Part print with two shaded views. Sizes in mm from the minimum x, y, z corner. A direction names the side the tool comes from. Round coordinates to 2 decimals unless told otherwise and drop trailing zeros. Order: outer loops, then holes, each group sorted by start corner. A loop starts at its lowest first (then second) coordinate and runs counter-clockwise, first axis right, second up. Notation, with made-up numbers: (83, 57) -> (90, 57) arc R26 cw to (90, 78) -> close; hole circle Ø4 at (20.25, -9.75). An arc over 180 degrees is marked (long way). Answer as a JSON object with one key per item and string values.
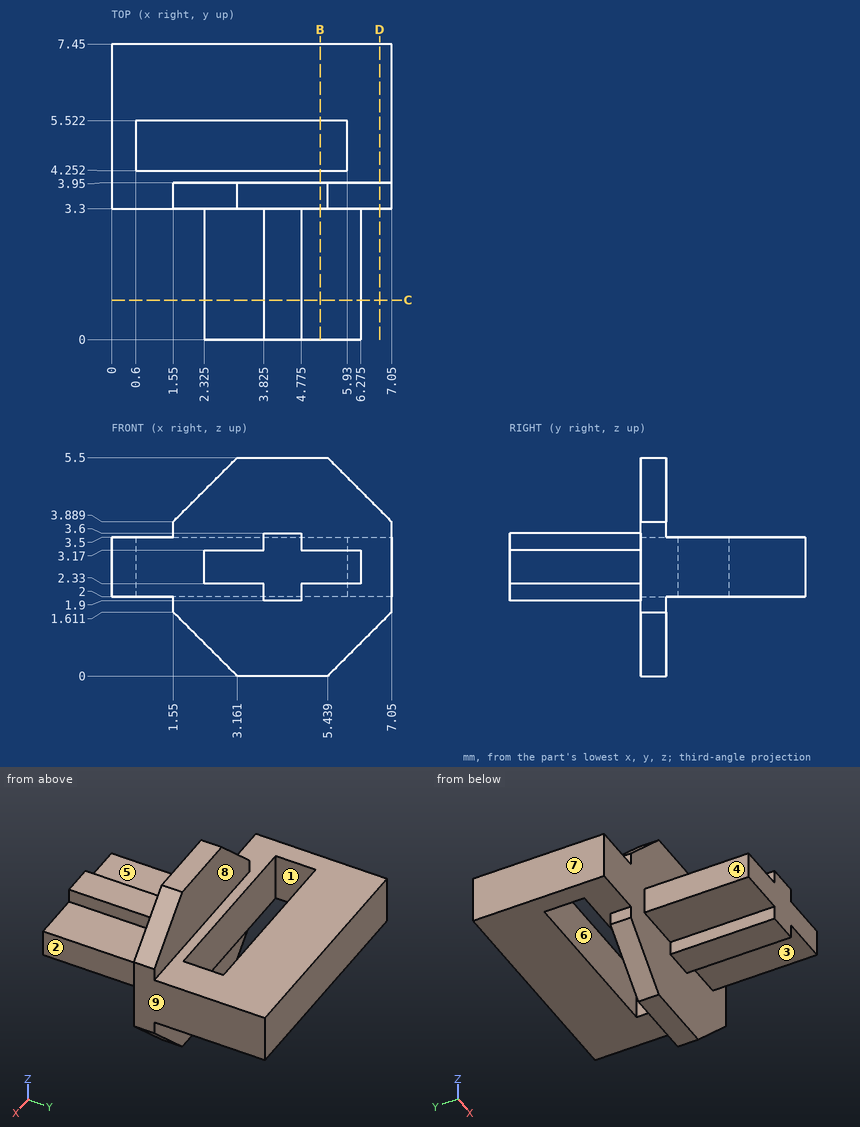
1) Cut at B-B, the plane x = 5.25. Give the cut face in (y, z).
Checked values:
{"outline": "(0, 2.33) -> (3.3, 2.33) -> (3.3, 0) -> (3.95, 0) -> (3.95, 2) -> (4.25, 2) -> (4.25, 3.5) -> (3.95, 3.5) -> (3.95, 5.5) -> (3.3, 5.5) -> (3.3, 3.17) -> (0, 3.17) -> close; (5.52, 2) -> (7.45, 2) -> (7.45, 3.5) -> (5.52, 3.5) -> close"}
2) Cut at C-C, the plane y = 1. Give the cut face in (x, z) (1 decimal).
Checked values:
{"outline": "(2.3, 2.3) -> (3.8, 2.3) -> (3.8, 1.9) -> (4.8, 1.9) -> (4.8, 2.3) -> (6.3, 2.3) -> (6.3, 3.2) -> (4.8, 3.2) -> (4.8, 3.6) -> (3.8, 3.6) -> (3.8, 3.2) -> (2.3, 3.2) -> close"}
3) Cut at D-D, the plane x = 6.75. Give the cut face in (y, z).
Checked values:
{"outline": "(3.3, 1.31) -> (3.95, 1.31) -> (3.95, 2) -> (7.45, 2) -> (7.45, 3.5) -> (3.95, 3.5) -> (3.95, 4.19) -> (3.3, 4.19) -> close"}
4) Flat gauge pins, fed straight in: pin 1 Ø0.7 at (y, z) = (1.5, 2.5) entering from +X (1 decimal); pin 2 Ø0.6 at (x, z) = (4.5, 4.5) entering from +Y; pin 3 Ø0.9 at (y, z) = (2, 2.5) entering from -X (1 decimal). Where does each tip first touch, or does it go through?
Checked values:
{"pin 1": "stops at x = 6.3", "pin 2": "stops at y = 3.95", "pin 3": "stops at x = 2.3"}
5) Probe L1, parallel to Y at x = 0.75, z = 2.1; L2, parallel to Y at x = 3, z = 3.1; L3, parallel to Y at x = 6.5, z = 4.2. List the from-to ranges inside material, lowest first. Write a range as from..to.
Checked values:
{"L1": "y = 3.3..4.25, 5.52..7.45", "L2": "y = 0..4.25, 5.52..7.45", "L3": "y = 3.3..3.95"}
6) Which spindle directions (+Z, -Z, +X, -X, +Y, -Y) get a long thin tool onto all of the face, cutting with end or side? Do the marked faces 1, 2, 3, 4 and 5. Say none if no direction does.
Checked values:
{"face 1": "+Z, -Z", "face 2": "+Z, -Z, +X, -Y", "face 3": "-Z, +X, -Y", "face 4": "+Z, -Z, -X, -Y", "face 5": "+Z, -X, -Y"}
7) Pull direction X, two halves, no side cores. Call the marked faces 6, 7, 8 and 9: pulls with the +X half, pulls with the -X half, needs draft (parallel to the pull), parting line crosses it, or undercut.
Checked values:
{"face 6": "undercut", "face 7": "pulls with the -X half", "face 8": "needs draft", "face 9": "pulls with the +X half"}
